from build123d import *
from build123d.topology import SkipClean

# Parameters (mm, degrees)
BOSS_EXTRUDE1_DEPTH = 7
SKETCH3_R           = 1
CUT_EXTRUDE1_DEPTH  = 10
RIB1_REACH          = 27.202
SKETCH2_WALL_W      = 65.053025346
SKETCH2_WALL_H      = 3
BOSS_EXTRUDE2_DEPTH = 7
SKETCH5_R           = 1
CUT_EXTRUDE2_DEPTH  = 14
FILLET1_R           = 1
FILLET2_R           = 0.4
SKETCH6_W           = 2
SKETCH6_H           = 4.221802259
CUT_EXTRUDE3_DEPTH  = 28.966741934
SKETCH7_W           = 1
SKETCH7_H           = 18.119739654
CUT_EXTRUDE4_DEPTH  = 28.966741934


with BuildPart() as part:
    # Sketch1 → Boss-Extrude1 (new, symmetric)
    with BuildSketch(Plane.XY):
        with BuildLine():
            Line((0, 10), (0, 7))
            ThreePointArc((0, 7), (7, 0), (0, -7))
            Line((0, -7), (0, -10))
            ThreePointArc((0, -10), (3.780589618, -9.257815193), (7, -7.141428429))
            Line((7, -7.141428429), (7, -19.751927866))
            Line((7, -19.751927866), (14, -19.751927866))
            Line((14, -19.751927866), (14, -16.751927866))
            Line((14, -16.751927866), (10, -16.751927866))
            Line((10, -16.751927866), (10, 0))
            ThreePointArc((10, 0), (7.071067812, 7.071067812), (0, 10))
        make_face()
    extrude(amount=BOSS_EXTRUDE1_DEPTH, both=True)

    # Sketch3 → Cut-Extrude1 (cut)
    with BuildSketch(Plane(origin=(0, -16.751927866, 0), x_dir=(1, 0, 0), z_dir=(0, 1, 0))):
        with Locations(Location((12, -4.2, 0), (0, 0, 270))):
            Circle(SKETCH3_R)
        with Locations(Location((12, 4.2, 0), (0, 0, 270))):
            Circle(SKETCH3_R)
    extrude(amount=-CUT_EXTRUDE1_DEPTH, mode=Mode.SUBTRACT)

    # Sketch2 wall → Rib1 (add, up to next)
    with BuildSketch(Plane(origin=(12, -10.751927866, 0), x_dir=(-0.316227766017, 0.948683298051, 0), z_dir=(-0.948683298051, -0.316227766017, 0)), mode=Mode.PRIVATE) as rib1_sk1:
        Rectangle(SKETCH2_WALL_W, SKETCH2_WALL_H)
    rib1_tool1 = extrude(rib1_sk1.sketch, amount=RIB1_REACH, mode=Mode.PRIVATE) - part.part
    add(rib1_tool1.solids().sort_by_distance((12, -10.751927866, 0))[0])

    # Sketch4 → Boss-Extrude2 (add, symmetric)
    with BuildSketch(Plane.XY):
        with BuildLine():
            Line((0, 10), (0, 13.139392014))
            Line((0, 13.139392014), (3, 13.139392014))
            Line((3, 13.139392014), (3, 9.539392014))
            ThreePointArc((3, 9.539392014), (1.517576993, 9.884177258), (0, 10))
        make_face()
    extrude(amount=BOSS_EXTRUDE2_DEPTH, both=True)

    # Sketch5 → Cut-Extrude2 (cut)
    with BuildSketch(Plane(origin=(3, 0, 0), x_dir=(0, 0, -1), z_dir=(1, 0, 0))):
        with Locations((-3.75, 11.339392014)):
            Circle(SKETCH5_R)
        with Locations((0, 11.339392014)):
            Circle(SKETCH5_R)
        with Locations((3.75, 11.339392014)):
            Circle(SKETCH5_R)
    extrude(amount=-CUT_EXTRUDE2_DEPTH, mode=Mode.SUBTRACT)

    # Fillet1
    fillet1_edges = [part.edges().sort_by_distance(p)[0] for p in [
        (3, 9.539392014, 0),
    ]]
    fillet(fillet1_edges, radius=FILLET1_R)

    # Fillet2
    fillet2_edges = [part.edges().sort_by_distance(p)[0] for p in [
        (1.5, 13.139392014, -7),
        (1.5, 13.139392014, 7),
    ]]
    fillet(fillet2_edges, radius=FILLET2_R)

    # Sketch6 → Cut-Extrude3 (cut, through all)
    with BuildSketch(Plane.XY.offset(7)):
        with Locations((8, -19.862828996)):
            Rectangle(SKETCH6_W, SKETCH6_H)
    extrude(amount=-CUT_EXTRUDE3_DEPTH, mode=Mode.SUBTRACT)

    # Mirror1: part across plane


with BuildPart() as part_1:
    with SkipClean():  # the faces are left unmerged after this step: merging them gives an invalid solid
        add(part.part)
        add(part.part.mirror(Plane(origin=(0, 0, 0), x_dir=(0, 0, 1), z_dir=(1, 0, 0))))

    # Sketch7 → Cut-Extrude4 (cut, through all)
    with BuildSketch(Plane.XY.offset(7)):
        with Locations((0, 9.869696007)):
            Rectangle(SKETCH7_W, SKETCH7_H)
    extrude(amount=-CUT_EXTRUDE4_DEPTH, mode=Mode.SUBTRACT)


solid = part_1.part
Geometry check sheet. Reference: the model listing, model coordinates, mm. A direction names the side the tool comes from. Round coordinates to 2 decimals unless told otherwise and drop trailing zeros. Loops run counter-clockwise (first coordinate to the right, second up) from the corner with the lowest first, then second, coordinate; pieces in that order, holes last.
Item 1: Cross-section at B-B on y = -9.5. Record the boundary of the cut face in (x, z), then the cut area to 3 significant figures.
Item 2: Gauge pin test, flat ends, axial feed: pin 1 (1.2 mm diameter, centred on x = 11.5, z = 3, fed in from +Y); pin 2 (1.6 mm diameter, centred on x = -12, z = 4.2, fed in from -Y); pin 3 (6 mm diameter, centred on x = -11, z = -5, fed in from +Y); pin 4 (4 mm diameter, centred on x = 11, z = 0.5, fed in from +Y). Record the tip position at first contact, or that the pin passes through.
Item 3: Thickness scan on line 1 (Z direction, x = -12, y = -18.1); line 2 (X direction, y = -18.6, z = 4.2); line 3 (X direction, y = -16, z = -2). Record the ranges inside material, lowest first.
Item 4: Access from +Z, -Z, +X, -X, +Y, -Y to the whole of each face (thin tool, end or side, straight path). Record for faces 1 (the flat face through (11, -16.752, 5)), 2 (the flat face through (3, 12.7, 0.1)), 3 (the flat face through (-10, -8, 2)), 4 (the flat face through (0.5, 10, 0)), 5 (the flat face through (-11, -16.752, -5)).
Item 5: Cross-section at D-D on x = 4. Record the boundary of the cut face in (y, z).
Item 6: Cross-section at C-C on x = -12. Record the boundary of the cut face in (y, z), then the cut area to 3 significant figures.
Item 7: Cross-section at A-A on x = -1.75. Record the boundary of the cut face in (y, z).
Item 8: Mould release check, pull along Z, two halves, no side actions. Record for faces 6 (the cylindrical face through (1.768, 10.731, -2.956)), 7 (the flat face through (1, -8, -7)), 8 (the flat face through (-8, -17.752, 0)): pulls with the +Z half, pulls with the -Z half, needs draft (parallel to the pull), parting line crosses it, or undercut.
Answer sheet:
1. outline: (-11.58, -1.5) - (-10, -1.5) - (-10, -7) - (-7, -7) - (-7, 7) - (-10, 7) - (-10, 1.5) - (-11.58, 1.5) - close; (-3.12, -7) - (3.12, -7) - (3.12, 7) - (-3.12, 7) - close; (7, -7) - (10, -7) - (10, -1.5) - (11.58, -1.5) - (11.58, 1.5) - (10, 1.5) - (10, 7) - (7, 7) - close
1. area: 181 mm2
2. pin 1: stops at y = -16.75
2. pin 2: passes through
2. pin 3: stops at y = 6
2. pin 4: stops at y = 4.36
3. line 1: z = -7 to -5.2, -3.2 to 3.2, 5.2 to 7
3. line 2: x = -14 to -13, -11 to -9, 9 to 11, 13 to 14
3. line 3: x = -10 to -7, 7 to 10
4. face 1: +Z, +X, +Y
4. face 2: +Z, -Z, +X, +Y
4. face 3: -X, +Y
4. face 4: +Z, -Z, +Y
4. face 5: -Z, -X, +Y
5. outline: (-9.17, -7) - (-5.74, -7) - (-5.74, 7) - (-9.17, 7) - close; (5.74, -7) - (9.17, -7) - (9.17, 7) - (5.74, 7) - close
6. outline: (-19.75, -7) - (-16.75, -7) - (-16.75, -5.2) - (-19.75, -5.2) - close; (-19.75, -3.2) - (-16.75, -3.2) - (-16.75, -1.5) - (-10.75, -1.5) - (-10.75, 1.5) - (-16.75, 1.5) - (-16.75, 3.2) - (-19.75, 3.2) - close; (-19.75, 5.2) - (-16.75, 5.2) - (-16.75, 7) - (-19.75, 7) - close
6. area: 48.0 mm2
7. outline: (-9.85, -7) - (-6.78, -7) - (-6.78, 7) - (-9.85, 7) - close; (6.78, -7) - (12.74, -7) arc R0.4 ccw to (13.14, -6.6) - (13.14, 6.6) arc R0.4 ccw to (12.74, 7) - (6.78, 7) - close; hole circle Ø2 at (11.34, -3.75); hole circle Ø2 at (11.34, 0); hole circle Ø2 at (11.34, 3.75)
8. face 6: undercut
8. face 7: pulls with the -Z half
8. face 8: needs draft
